from build123d import *

# Parameters (mm, degrees)
BOSS_EXTRU_1_DEPTH      = 52
ESQUISSE4_W             = 351.485824357
ESQUISSE4_H             = 52
ENL_V_MAT_EXTRU_1_DEPTH = 52


with BuildPart() as part:
    # Esquisse3 → Boss.-Extru.1 (new body)
    with BuildSketch(Plane(origin=(0, 0, 0), x_dir=(1, 0, 0), z_dir=(0, 1, 0))):
        Polygon((341.486019825, 0), (0, 0), (-9.995686149, 0), (-9.999804532, -0.431819515), (0, -0.5), (220, -2), (341.486019825, -2), align=None)
    extrude(amount=BOSS_EXTRU_1_DEPTH)

    # Esquisse4 → Enlèv. mat.-Extru.1 (cut)
    with BuildSketch(Plane.XY.offset(2)):
        with Locations((165.743107647, 26)):
            Rectangle(ESQUISSE4_W, ESQUISSE4_H)
        with BuildLine():
            Line((325, 46.5), (325, 36))
            Line((325, 36), (220, 36))
            Line((220, 36), (220, 34.5))
            add(Edge.make_bspline(
                [(220, 34.5), (210.148627769, 34.5), (202, 34.902841403), (202, 21.363033151)],
                knots=[0, 0, 0, 0, 1, 1, 1, 1], degree=3))
            Line((202, 21.363033151), (202, 4))
            add(Edge.make_bspline(
                [(202, 4), (25.782341649, 14.763588637), (0, 34.373939813)],
                knots=[0, 0, 0, 1, 1, 1], degree=2))
            add(Edge.make_bspline(
                [(0, 34.373939813), (26.740576578, 53.810637401), (88.50602407, 48), (220, 48)],
                knots=[0, 0, 0, 0, 1, 1, 1, 1], degree=3))
            Line((220, 48), (220, 46.5))
            Line((220, 46.5), (325, 46.5))
        make_face(mode=Mode.SUBTRACT)
    extrude(amount=-ENL_V_MAT_EXTRU_1_DEPTH, mode=Mode.SUBTRACT)


solid = part.part
CAD build for the part. Positions are in the model's coordinates, mm. Coordinates: 2 decimals unless noted, no trailing zeros. Order: outer loops, then holes, each group sorted by start corner. A loop starts at its lowest first (then second) coordinate and runs counter-clockwise, first axis right, second up.
Item 1: Pin check, flat tips, straight feed: pin 1 Ø6 at (x, y) = (258, 34) entering from -Z; pin 2 Ø1 at (x, y) = (172.5, 19) entering from +Z; pin 3 Ø0.8 at (y, z) = (35.5, 1) entering from +X. Stop position of each tip, or through.
Check sheet entries:
pin 1: stops at z = 0
pin 2: stops at z = 1.68
pin 3: stops at x = 220
Item 2: Band-saw the part on A-A on x = 243. List the corners of the cut face in (y, z).
Check sheet entries:
outline: (36, 0) - (46.5, 0) - (46.5, 2) - (36, 2) - close
Item 3: Drill centre lines: L1, parallel to Y at x = 267, z = 0.5; L2, parallel to Y at x = 140.5, z = 1.1; L3, parallel to Z at x = 166, y = 15. Where is each one in solid material? Low to high.
Check sheet entries:
L1: y = 36 to 46.5
L2: y = 8.41 to 48.54
L3: z = 0 to 1.63
